Can you work these out from the model? Positions are in its coordinate system, mm. Face numbers are marked on the shaded views. A direction names the side the tool comes from. Coordinates: 2 decimals unless noted, no trailing zeros. Order: outer loops, then holes, each group sorted by start corner. A loop starts at its lowest first (then second) coordinate and runs counter-clockwise, first axis right, second up. Notation, with made-up numbers: M 28,60 L 71,60 A18 cw 71,90 Z; hole C 20.5,68.25 d10. An arc over 180 degrees is marked long. Answer as a JSON object with one key per item and string values.
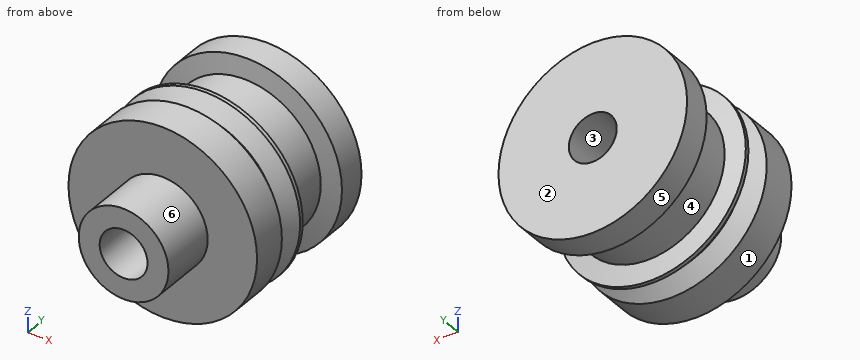
Autodesk Inventor part; units mm, degrees
ref_plane "YZ Plane" through (0, 0, 0) normal (1, 0, 0) x (0, 1, 0)
ref_plane "XZ Plane" through (0, 0, 0) normal (0, 1, 0) x (-1, 0, 0)
ref_plane "XY Plane" through (0, 0, 0) normal (0, 0, 1) x (1, 0, 0)
sketch "Sketch1" plane through (0, 0, 0) normal (0, 0, 1) x (1, 0, 0)
  line L0 (0, 0) -> (0, 17.163)
  line L1 (2.5, 4) -> (2.5, 3.25)
  line L2 (2.5, 0) -> (0, 0)
  line L3 (2.5, 3.25) -> (2, 3.1618)
  line L4 (2, 3.1618) -> (2, 1.8382)
  line L5 (2, 1.8382) -> (2.5, 1.75)
  line L6 (0, 0) -> (0, 4)
  line L7 (0, 4) -> (2.5, 4)
  line L8 (2.5, 1.65) -> (2.15, 1.3)
  line L9 (2.15, 1.3) -> (2.5, 0.95)
  line L10 (2.5, 1.75) -> (2.5, 1.65)
  line L11 (2.5, 0.95) -> (2.5, 0)
  dimension "d2" = 5
  dimension "d17" = 0.75
  dimension "d18" = 1.75
  dimension "d19" = 100
  dimension "d20" = 100
  dimension "d24" = 1.3237
  dimension "d53" = 1.3
  dimension "d54" = 135
  dimension "d55" = 135
  dimension "d56" = 0.35
revolve "Revolution1" add sketch "Sketch1" angle 360 about axis through (0, 0, 0) along (0, 1, 0)
hole "Hole1" [suppressed]
sketch "Sketch2" plane through (0, 0, 0) normal (0, -1, 0) x (1, 0, 0)
  circle A0 centre (0, 0) radius 1.19
  dimension "d36" = 2.38
extrude "Extrusion1" add sketch "Sketch2" along normal blind 1.5
hole "Hole3" at (0, -1.5, 0) direction (0, 1, 0) diameter 1.27 end through all
properties part number "FOX-ME-126-05" material "CU 110H04"
Item 1: I'm going to push a flat-ended pin straight in: pin 1 (1.5 mm diameter, centred on x = 0.5, y = 2, fed in from +Z). Where does the tip first touch, or does it pass through?
Answers follow:
{"pin 1": "stops at z = 2.5"}
Item 2: Which directions (+Z, -Z, +X, -X, +Y, -Y) give clear straight access to the entire face, cutting with the end or side of a thin tool? Please do the marked faces 4, 5 and 6.
Answers follow:
{"face 4": "none", "face 5": "+Y, -Y", "face 6": "-Y"}
Item 3: I want a section at B-B, the plane x = 0. Write out the boundary of the cut face in (y, z) (3 decimals), plus the area to 3 significant figures.
Answers follow:
{"outline": "M -1.5,-1.19 L 0,-1.19 L 0,-2.5 L 0.95,-2.5 L 1.3,-2.15 L 1.65,-2.5 L 1.75,-2.5 L 1.838,-2 L 3.162,-2 L 3.25,-2.5 L 4,-2.5 L 4,-0.635 L -1.5,-0.635 Z; M -1.5,0.635 L 4,0.635 L 4,2.5 L 3.25,2.5 L 3.162,2 L 1.838,2 L 1.75,2.5 L 1.65,2.5 L 1.3,2.15 L 0.95,2.5 L 0,2.5 L 0,1.19 L -1.5,1.19 Z", "area": "14.9 mm^2"}
Item 4: If we mould it in two halves opening along Z, with no side actions, what happens to the marked faces 1, 2 and 3? For each: pulls with the +Z half, pulls with the -Z half, needs draft (parallel to the pull), parting line crosses it, or undercut.
Answers follow:
{"face 1": "parting line crosses it", "face 2": "needs draft", "face 3": "undercut"}
Item 5: I want a section at A-A, the plane z = 0. Write out the boundary of the cut face in (x, y) (3 decimals).
Answers follow:
{"outline": "M -2.5,0 L -1.19,0 L -1.19,-1.5 L -0.635,-1.5 L -0.635,4 L -2.5,4 L -2.5,3.25 L -2,3.162 L -2,1.838 L -2.5,1.75 L -2.5,1.65 L -2.15,1.3 L -2.5,0.95 Z; M 0.635,-1.5 L 1.19,-1.5 L 1.19,0 L 2.5,0 L 2.5,0.95 L 2.15,1.3 L 2.5,1.65 L 2.5,1.75 L 2,1.838 L 2,3.162 L 2.5,3.25 L 2.5,4 L 0.635,4 Z"}
Item 6: Please list where these lines run through material, in increasing order: line 1 (X direction, y = 2.8, z = 0.05); line 2 (Y direction, x = 2.15, z = -0.75); line 3 (X direction, y = 0.9, z = 0) (3 decimals).
Answers follow:
{"line 1": "x = -2 to -0.63, 0.63 to 2", "line 2": "y = 0 to 1.17, 1.43 to 1.79, 3.21 to 4", "line 3": "x = -2.5 to -0.635, 0.635 to 2.5"}
